Could you check a few things on this model? Use its own coordinates, in mm. A direction names the side the tool comes from. Give positions to 0.01 mm unless a question says otherwise; leave off trailing zeros. Loops run counter-clockwise (first coordinate to the right, second up) from the corner with the lowest first, then second, coordinate; pieces in that order, holes last. Notation, with made-up numbers: (4.5, -17.5) -> (13.5, -17.5) arc R11 ccw to (13.5, -10.5) -> close; hole circle Ø1 at (59, -14). An arc over 180 degrees is marked (long way). Write item = value, one per line. Start each with the question number.
1) I need wall thicknesses on probe 1 along Y at (x, z) = (10.5, -19.65); probe 2 along Y at (x, z) = (-10.5, -17.4); probe 3 along X at (y, z) = (7.5, -1). Which ranges of each line are inside material? Lowest first, please. Write a range as from..to.
2) On a 3-axis mill with a long thin cutter (end or side, diameter ignored), from which of +Z, -Z, +X, -X, +Y, -Y can I reach the whole of each face in a straight line? I mean faces 3 (the face through (-11.49, 21.74, -17.96)), 4 (the face through (-10.21, 37.23, -19.77)), 5 (the face through (19.014, 32.855, -12.552)), 6 (the face through (16.36, 1.52, -7.98)), 7 (the face through (4, 24, -15)). Say none if no direction works.
3) I want a section at B-B (z = 5). List the corners of the cut face in (x, y) for me, and give its area (3 significant figures).
4) I want a section at A-A (y = 22.5). List the corners of the cut face in (x, z) for me.
5) If we mould it in two halves opening along X, with no side actions, what happens to faces 1 (the face through (-9.5, 23.5, -21)), 2 (the face through (-16.36, 1.52, -5.02))? For each: +X half, -X half, draft (parallel to the pull), parting line (faces both ways), or undercut.
6) I want a section at C-C (z = -5). List the corners of the cut face in (x, y) for me, and give its area (3 significant figures).
7) I'm going to push flat-ended pins straight in: pin 1 Ø1.5 at (x, z) = (0.5, 3.5) entering from +Y; pin 2 Ø4 at (y, z) = (19.5, 1) entering from -X; pin 3 Ø1 at (x, y) = (7, 21.5) entering from +Z; pin 4 Ø8 at (x, y) = (-14.5, 12) entering from +Z. Where does each tip first touch, or does it pass through?
8) I want a section at D-D (x = -6). List the corners of the cut face in (y, z) for me, and give its area (4 significant figures).
from build123d import *

# Parameters (mm, degrees)
SKETCH1_W             = 40
SKETCH1_H             = 30
BOSS_EXTRUDE1_DEPTH   = 3
CUT_EXTRUDE1_REACH    = 27.179
SKETCH3_W             = 40
SKETCH3_H             = 6
BOSS_EXTRUDE2_DEPTH   = 45
RIB1_REACH            = 65.765
SKETCH5_WALL_W        = 171.255680626
SKETCH5_WALL_H        = 2
RIB2_START            = -2
RIB2_DEPTH            = 2
FILLET1_R             = 30
SKETCH7_W             = 30
SKETCH7_H             = 35
SKETCH7_R             = 2.25
CUT_EXTRUDE2_DEPTH    = 2.5
F_2_5MM_DOWEL_HOLE1_D = 2.5


# Read off the part's stored shape, not the designer's step: Rib2
with BuildPart() as part:
    # Sketch1 → Boss-Extrude1 (new body)
    with BuildSketch(Plane(origin=(0, 0, 0), x_dir=(1, 0, 0), z_dir=(0, 1, 0))):
        Rectangle(SKETCH1_W, SKETCH1_H)
    extrude(amount=BOSS_EXTRUDE1_DEPTH)

    # Sketch2 → Cut-Extrude1 (cut, up to next)
    with BuildSketch(Plane(origin=(0, 3, 0), x_dir=(1, 0, 0), z_dir=(0, 1, 0)), mode=Mode.PRIVATE) as cut_extrude1_sk1:
        Polygon((-10.285898385, 6.5), (-12.017949192, 9.5), (-15.482050808, 9.5), (-17.214101615, 6.5), (-15.482050808, 3.5), (-12.017949192, 3.5), align=None)
    cut_extrude1_tool1 = extrude(cut_extrude1_sk1.sketch, amount=-CUT_EXTRUDE1_REACH, mode=Mode.PRIVATE) & part.part
    # Sketch2 → Cut-Extrude1 (cut, up to next)
    with BuildSketch(Plane(origin=(0, 3, 0), x_dir=(1, 0, 0), z_dir=(0, 1, 0)), mode=Mode.PRIVATE) as cut_extrude1_sk2:
        Polygon((17.214101615, 6.5), (15.482050808, 9.5), (12.017949192, 9.5), (10.285898385, 6.5), (12.017949192, 3.5), (15.482050808, 3.5), align=None)
    cut_extrude1_tool2 = extrude(cut_extrude1_sk2.sketch, amount=-CUT_EXTRUDE1_REACH, mode=Mode.PRIVATE) & part.part
    # Sketch2 → Cut-Extrude1 (cut, up to next)
    with BuildSketch(Plane(origin=(0, 3, 0), x_dir=(1, 0, 0), z_dir=(0, 1, 0)), mode=Mode.PRIVATE) as cut_extrude1_sk3:
        Polygon((-1.732050808, -9.5), (1.732050808, -9.5), (3.464101615, -6.5), (1.732050808, -3.5), (-1.732050808, -3.5), (-3.464101615, -6.5), align=None)
    cut_extrude1_tool3 = extrude(cut_extrude1_sk3.sketch, amount=-CUT_EXTRUDE1_REACH, mode=Mode.PRIVATE) & part.part
    add(cut_extrude1_tool1.solids().sort_by_distance((-13.75, 3, -6.5))[0], mode=Mode.SUBTRACT)
    add(cut_extrude1_tool2.solids().sort_by_distance((13.75, 3, -6.5))[0], mode=Mode.SUBTRACT)
    add(cut_extrude1_tool3.solids().sort_by_distance((0, 3, 6.5))[0], mode=Mode.SUBTRACT)

    # Sketch3 → Boss-Extrude2 (add)
    with BuildSketch(Plane.XZ):
        with Locations((0, -18)):
            Rectangle(SKETCH3_W, SKETCH3_H)
    extrude(amount=-BOSS_EXTRUDE2_DEPTH)

    # Sketch5 wall → Rib1 (add, up to next)
    with BuildSketch(Plane(origin=(-20, 17.5, 0), x_dir=(0, -0.695022096847, 0.718988376049), z_dir=(0, 0.718988376049, 0.695022096847)), mode=Mode.PRIVATE) as rib1_sk1:
        with Locations((0, 1)):
            Rectangle(SKETCH5_WALL_W, SKETCH5_WALL_H)
    rib1_tool1 = extrude(rib1_sk1.sketch, amount=-RIB1_REACH, mode=Mode.PRIVATE) - part.part
    add(rib1_tool1.solids().sort_by_distance((-20, 17.5, 0))[0])

    # Rib2 outline → Rib2 (add)
    with BuildSketch(Plane(origin=(20, 0, 0), x_dir=(0, 0, -1), z_dir=(1, 0, 0)).offset(RIB2_START)):
        Polygon((15, 32), (-15, 3), (15, 3), align=None)
    extrude(amount=RIB2_DEPTH)

    # Fillet1
    fillet1_edges = [part.edges().sort_by_distance(p)[0] for p in [
        (19, 32, -15),
        (-19, 32, -15),
    ]]
    fillet(fillet1_edges, radius=FILLET1_R)

    # Sketch7 → Cut-Extrude2 (cut)
    with BuildSketch(Plane(origin=(0, 0, -21), x_dir=(-1, 0, 0), z_dir=(0, 0, -1))):
        with Locations((0, 22.5)):
            Rectangle(SKETCH7_W, SKETCH7_H)
        with Locations((-10.5, 35)):
            Circle(SKETCH7_R, mode=Mode.SUBTRACT)
        with Locations((10.5, 35)):
            Circle(SKETCH7_R, mode=Mode.SUBTRACT)
        with Locations((10.5, 22.5)):
            Circle(SKETCH7_R, mode=Mode.SUBTRACT)
        with Locations((-10.5, 22.5)):
            Circle(SKETCH7_R, mode=Mode.SUBTRACT)
    extrude(amount=-CUT_EXTRUDE2_DEPTH, mode=Mode.SUBTRACT)

    # Ø2.5mm Dowel Hole1 (through all)
    with Locations(Plane(origin=(0, 0, -21), x_dir=(-1, 0, 0), z_dir=(0, 0, -1))):
        with Locations((10.5, 35), (-10.5, 35), (-10.5, 22.5), (10.5, 22.5)):
            Hole(F_2_5MM_DOWEL_HOLE1_D / 2)


solid = part.part
Answer list:
q1.probe_1 = 0..5, 20.25..21.25, 23.75..24.75, 32.75..33.75, 36.25..37.25, 40..45
q1.probe_2 = 0..21.25, 23.75..33.75, 36.25..45
q1.probe_3 = -20..-18, 18..20
q2.face_3 = +Z, -Z
q2.face_4 = -Z
q2.face_5 = +Z, +X, -X, +Y
q2.face_6 = +Y, -Y
q2.face_7 = +Z, +Y
q3.outline = (-20, 0) -> (-2.6, 0) -> (-2.6, 3) -> (-18, 3) -> (-18, 12.67) -> (-20, 12.67) -> close; (2.6, 0) -> (20, 0) -> (20, 12.67) -> (18, 12.67) -> (18, 3) -> (2.6, 3) -> close
q3.area = 143 mm^2
q4.outline = (-20, -21) -> (-15, -21) -> (-15, -18.5) -> (-12.75, -18.5) -> (-12.75, -21) -> (-11.75, -21) -> (-11.75, -15) -> (-18, -15) -> (-18, -5.17) -> (-20, -5.17) -> close; (-9.25, -21) -> (-8.25, -21) -> (-8.25, -18.5) -> (8.25, -18.5) -> (8.25, -21) -> (9.25, -21) -> (9.25, -15) -> (-9.25, -15) -> close; (11.75, -21) -> (12.75, -21) -> (12.75, -18.5) -> (15, -18.5) -> (15, -21) -> (20, -21) -> (20, -5.17) -> (18, -5.17) -> (18, -15) -> (11.75, -15) -> close
q5.face_1 = draft
q5.face_2 = undercut
q6.outline = (-20, 0) -> (-16.35, 0) -> (-16.35, 3) -> (-18, 3) -> (-18, 22.33) -> (-20, 22.33) -> close; (-11.15, 0) -> (11.15, 0) -> (11.15, 3) -> (-11.15, 3) -> close; (16.35, 0) -> (20, 0) -> (20, 22.33) -> (18, 22.33) -> (18, 3) -> (16.35, 3) -> close
q6.area = 166 mm^2
q7.pin_1 = 3
q7.pin_2 = through
q7.pin_3 = -15
q7.pin_4 = 7.69
q8.outline = (0, -21) -> (5, -21) -> (5, -18.5) -> (40, -18.5) -> (40, -21) -> (45, -21) -> (45, -15) -> (3, -15) -> (3, 15) -> (0, 15) -> close
q8.area = 272.5 mm^2
